from build123d import *

# Parameters (mm, degrees)
SKETCH1_R           = 2.5
BOSS_EXTRUDE1_DEPTH = 7.23
CUT_EXTRUDE1_START  = -6.43
CUT_EXTRUDE1_DEPTH  = 6.43
CUT_EXTRUDE2_START  = -13
SKETCH5_R           = 1.25
CUT_EXTRUDE2_DEPTH  = 13
BOSS_EXTRUDE2_DEPTH = 3.5
BOSS_EXTRUDE3_DEPTH = 2


with BuildPart() as part:
    # Sketch1 → Boss-Extrude1 (new body)
    with BuildSketch(Plane(origin=(0, 0, 0), x_dir=(1, 0, 0), z_dir=(0, 1, 0))):
        with BuildLine():
            Line((-8, -10), (8, -10))
            ThreePointArc((8, -10), (9.414213562, -9.414213562), (10, -8))
            Line((10, -8), (10, 8))
            ThreePointArc((10, 8), (9.414213562, 9.414213562), (8, 10))
            Line((8, 10), (-8, 10))
            ThreePointArc((-8, 10), (-9.414213562, 9.414213562), (-10, 8))
            Line((-10, 8), (-10, -8))
            ThreePointArc((-10, -8), (-9.414213562, -9.414213562), (-8, -10))
        make_face()
        with Locations(Location((3.5, 0, 0), (0, 0, 270))):
            Circle(SKETCH1_R, mode=Mode.SUBTRACT)
        with Locations(Location((-3.5, 0, 0), (0, 0, 270))):
            Circle(SKETCH1_R, mode=Mode.SUBTRACT)
    extrude(amount=BOSS_EXTRUDE1_DEPTH)

    # Sketch2 → Cut-Extrude1 (cut)
    with BuildSketch(Plane(origin=(0, 7.23, 0), x_dir=(1, 0, 0), z_dir=(0, 1, 0)).offset(CUT_EXTRUDE1_START)):
        with BuildLine():
            Line((3.25, 3), (3.25, 2.487468593))
            ThreePointArc((3.25, 2.487468593), (3.5, 2.5), (3.75, 2.487468593))
            Line((3.75, 2.487468593), (3.75, 3))
            Line((3.75, 3), (3.25, 3))
        make_face()
        with BuildLine():
            ThreePointArc((6, 0), (5.996865183, -0.125156938), (5.987468593, -0.25))
            Line((5.987468593, -0.25), (6.5, -0.25))
            Line((6.5, -0.25), (6.5, 0.25))
            Line((6.5, 0.25), (5.987468593, 0.25))
            ThreePointArc((5.987468593, 0.25), (5.996865183, 0.125156938), (6, 0))
        make_face()
        with BuildLine():
            Line((3.25, -2.487468593), (3.25, -3))
            Line((3.25, -3), (3.75, -3))
            Line((3.75, -3), (3.75, -2.487468593))
            ThreePointArc((3.75, -2.487468593), (3.5, -2.5), (3.25, -2.487468593))
        make_face()
        with BuildLine():
            Line((0.5, -0.25), (1.012531407, -0.25))
            ThreePointArc((1.012531407, -0.25), (1, 0), (1.012531407, 0.25))
            Line((1.012531407, 0.25), (0.5, 0.25))
            Line((0.5, 0.25), (0.5, -0.25))
        make_face()
        with BuildLine():
            ThreePointArc((-1, 0), (-1.003134817, -0.125156938), (-1.012531407, -0.25))
            Line((-1.012531407, -0.25), (-0.5, -0.25))
            Line((-0.5, -0.25), (-0.5, 0.25))
            Line((-0.5, 0.25), (-1.012531407, 0.25))
            ThreePointArc((-1.012531407, 0.25), (-1.003134817, 0.125156938), (-1, 0))
        make_face()
        with BuildLine():
            Line((-3.75, 3), (-3.75, 2.487468593))
            ThreePointArc((-3.75, 2.487468593), (-3.5, 2.5), (-3.25, 2.487468593))
            Line((-3.25, 2.487468593), (-3.25, 3))
            Line((-3.25, 3), (-3.75, 3))
        make_face()
        with BuildLine():
            Line((-6.5, 0.25), (-6.5, -0.25))
            Line((-6.5, -0.25), (-5.987468593, -0.25))
            ThreePointArc((-5.987468593, -0.25), (-6, 0), (-5.987468593, 0.25))
            Line((-5.987468593, 0.25), (-6.5, 0.25))
        make_face()
        with BuildLine():
            ThreePointArc((-3.25, -2.487468593), (-3.5, -2.5), (-3.75, -2.487468593))
            Line((-3.75, -2.487468593), (-3.75, -3))
            Line((-3.75, -3), (-3.25, -3))
            Line((-3.25, -3), (-3.25, -2.487468593))
        make_face()
    extrude(amount=CUT_EXTRUDE1_DEPTH, mode=Mode.SUBTRACT)

    # Sketch3 → Revolve1 (revolve)
    with BuildSketch(Plane(origin=(0, 0, 0), x_dir=(0, 0, -1), z_dir=(1, 0, 0)), mode=Mode.PRIVATE) as revolve1_sk:
        Polygon((-10, 0.6), (-13, 0.6), (-13, 0), (-15.5, 1), (-15.5, 1.5), (-10, 1.5), align=None)
    revolve(revolve1_sk.sketch.rotate(Axis((0, 2.75, 10), (0, 0, 1)), 180), axis=Axis((0, 2.75, 10), (0, 0, 1)))

    # Sketch5 → Cut-Extrude2 (cut)
    with BuildSketch(Plane.XY.offset(10).offset(CUT_EXTRUDE2_START)):
        with Locations(Location((0, 2.75, 0), (0, 0, 90))):
            Circle(SKETCH5_R)
    extrude(amount=CUT_EXTRUDE2_DEPTH, mode=Mode.SUBTRACT)

    # Sketch6 → Boss-Extrude2 (add)
    with BuildSketch(Plane(origin=(0, 7.23, 0), x_dir=(1, 0, 0), z_dir=(0, 1, 0))):
        with BuildLine():
            Line((-8, -10), (8, -10))
            ThreePointArc((8, -10), (9.414213562, -9.414213562), (10, -8))
            Line((10, -8), (10, 8))
            ThreePointArc((10, 8), (9.414213562, 9.414213562), (8, 10))
            Line((8, 10), (-8, 10))
            ThreePointArc((-8, 10), (-9.414213562, 9.414213562), (-10, 8))
            Line((-10, 8), (-10, -8))
            ThreePointArc((-10, -8), (-9.414213562, -9.414213562), (-8, -10))
        make_face()
        with BuildLine():
            Line((-5, -7), (5, -7))
            ThreePointArc((5, -7), (6.414213562, -6.414213562), (7, -5))
            Line((7, -5), (7, 5))
            ThreePointArc((7, 5), (6.414213562, 6.414213562), (5, 7))
            Line((5, 7), (-5, 7))
            ThreePointArc((-5, 7), (-6.414213562, 6.414213562), (-7, 5))
            Line((-7, 5), (-7, -5))
            ThreePointArc((-7, -5), (-6.414213562, -6.414213562), (-5, -7))
        make_face(mode=Mode.SUBTRACT)
    extrude(amount=BOSS_EXTRUDE2_DEPTH)

    # Sketch8 → Boss-Extrude3 (add)
    with BuildSketch(Plane(origin=(0, 10.73, 0), x_dir=(1, 0, 0), z_dir=(0, 1, 0))):
        with BuildLine():
            Line((-8, -10), (8, -10))
            ThreePointArc((8, -10), (9.414213562, -9.414213562), (10, -8))
            Line((10, -8), (10, 8))
            ThreePointArc((10, 8), (9.414213562, 9.414213562), (8, 10))
            Line((8, 10), (-8, 10))
            ThreePointArc((-8, 10), (-9.414213562, 9.414213562), (-10, 8))
            Line((-10, 8), (-10, -8))
            ThreePointArc((-10, -8), (-9.414213562, -9.414213562), (-8, -10))
        make_face()
        with BuildLine():
            Line((-7, -9), (7, -9))
            ThreePointArc((7, -9), (8.414213562, -8.414213562), (9, -7))
            Line((9, -7), (9, 7))
            ThreePointArc((9, 7), (8.414213562, 8.414213562), (7, 9))
            Line((7, 9), (-7, 9))
            ThreePointArc((-7, 9), (-8.414213562, 8.414213562), (-9, 7))
            Line((-9, 7), (-9, -7))
            ThreePointArc((-9, -7), (-8.414213562, -8.414213562), (-7, -9))
        make_face(mode=Mode.SUBTRACT)
    extrude(amount=BOSS_EXTRUDE3_DEPTH)


solid = part.part
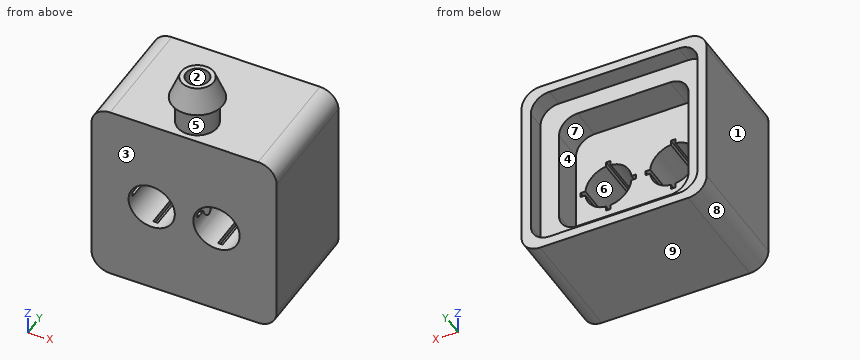
The listing builds one solid part. Answer for the finished solid, in the listing's coordinates (mm). Face numbers are marked on the shaded views. A direction names the side the tool comes from. Coordinates: 2 decimals unless noted, no trailing zeros. Loops run counter-clockwise (first coordinate to the right, second up) from the corner with the lowest first, then second, coordinate; pieces in that order, holes last. Notation, with made-up numbers: (72.5, 46) -> (91.5, 46) arc R34 ccw to (91.5, 80) -> close; hole circle Ø5 at (68, 66). An arc over 180 degrees is marked (long way). Write item = value, one per line. Start each with the question number.
1) A cutting plane is placed at C-C (x = 5.5). Give the vertices of the cut face in (y, z).
2) The mould has two halves that part along X. Classify the marked faces 6, 7, 8 and 9: released by +X, released by -X, zero draft, split by the parting line, or undercut.
3) A cutting plane is placed at B-B (y = 11.25). Give the vertices of the cut face in (x, z).
4) A cutting plane is placed at D-D (z = 6). Give the vertices of the cut face in (x, y), then the cut area to 3 significant figures.
5) Straight lines are drawn through the part: line 1 (X direction, y = 4.5, z = 0); line 2 (X direction, y = 2.75, z = 7); line 3 (Z direction, x = 3.5, y = 4). For each, find the intervals that lie inside material, in ascending order. Write a range as from..to.
6) A cutting plane is placed at A-A (z = -2). Give the vertices of the cut face in (x, y), then the cut area to 3 significant figures.
7) A tool of negligible diameter and unlimited length cuts with its end or side. For the marked faces 1, 2, 3, 4 and 5, from which of +Z, -Z, +X, -X, +Y, -Y can it reach the whole face along a straight path? Write none if from no direction.
8) Given pin 1 Ø3 at (x, z) = (0.5, -5.5) entering from -Y; pin 2 Ø1.5 at (y, z) = (10, 9.5) entering from -X; pin 3 Ø4 at (x, y) = (-7, 4.5) entering from +Z; pin 4 Ø0.6 at (x, z) = (3.5, 3) entering from +Y, each flat-ended and moving along its own axis, determine where each tip first touches the part or whether it passes through.
Responses:
q1.outline = (0, -10) -> (12.73, -10) -> (12.73, -9) -> (10.73, -9) -> (10.73, -6.94) -> (7.23, -6.94) -> (7.23, -1.5) -> (0, -1.5) -> close; (0, 1.5) -> (7.23, 1.5) -> (7.23, 6.94) -> (10.73, 6.94) -> (10.73, 9) -> (12.73, 9) -> (12.73, 10) -> (0, 10) -> close
q2.face_6 = undercut
q2.face_7 = undercut
q2.face_8 = released by -X
q2.face_9 = zero draft
q3.outline = (-10, -8) arc R2 ccw to (-8, -10) -> (8, -10) arc R2 ccw to (10, -8) -> (10, 8) arc R2 ccw to (8, 10) -> (-8, 10) arc R2 ccw to (-10, 8) -> close; hole (-9, -7) arc R2 ccw to (-7, -9) -> (7, -9) arc R2 ccw to (9, -7) -> (9, 7) arc R2 ccw to (7, 9) -> (-7, 9) arc R2 ccw to (-9, 7) -> close
q4.outline = (-10, 0) -> (10, 0) -> (10, 12.73) -> (9, 12.73) -> (9, 10.73) -> (6.73, 10.73) -> (6.73, 7.23) -> (-6.73, 7.23) -> (-6.73, 10.73) -> (-9, 10.73) -> (-9, 12.73) -> (-10, 12.73) -> close; hole circle Ø2.5 at (0, 2.75)
q4.area = 167 mm²
q5.line_1 = -10..-6.5, -0.5..0.5, 6.5..10
q5.line_2 = -10..-1.25, 1.25..10
q5.line_3 = -10..-3, 3..10
q6.outline = (-10, 0) -> (-5, 0) -> (-5, 7.23) -> (-7, 7.23) -> (-7, 10.73) -> (-9, 10.73) -> (-9, 12.73) -> (-10, 12.73) -> close; (-2, 0) -> (2, 0) -> (2, 7.23) -> (-2, 7.23) -> close; (5, 0) -> (10, 0) -> (10, 12.73) -> (9, 12.73) -> (9, 10.73) -> (7, 10.73) -> (7, 7.23) -> (5, 7.23) -> close; hole circle Ø2.5 at (0, 2.75)
q6.area = 121 mm²
q7.face_1 = +Z, -Z, -X, +Y, -Y
q7.face_2 = +Z
q7.face_3 = +Z, -Z, +X, -X, -Y
q7.face_4 = +Y
q7.face_5 = none
q8.pin_1 = 0
q8.pin_2 = -9.85
q8.pin_3 = 10
q8.pin_4 = 7.23
